Read the model definition and answer for the solid it produces. Units are mm, in the model's axes. Face numbers are marked on the shaded views. A direction names the side the tool comes from. Give positions to 0.01 mm unless a question says otherwise; leave off trailing zeros. Loops run counter-clockwise (first coordinate to the right, second up) from the corner with the lowest first, then second, coordinate; pieces in that order, holes last.
(1) Find section C-C, the plane z = 9. Write down the section's boundary in (x, y), then the cut area to 3 significant figures.
(2) Find section A-A, the plane x = -4. Write down the section's boundary in (y, z), then the cut area to 3 significant figures.
(3) Find section D-D, the plane y = 9.5. Write down the section's boundary in (x, z).
(4) Each of these flat-tipped pins is pushed along its axis until it touches: P1, Ø8, axis at y = 31, z = -1, coming from the -X side; P2, Ø5, axis at y = 30.5, z = 0, coming from the +X side; P3, Ø1, axis at x = -3, y = 29, coming from the -Z side. Where does it stop, or does it pass through?
(5) Straight lines are drawn through the part: probe 1 along X at (y, z) = (11.5, 0); probe 2 along Z at (x, y) = (-3.25, 31); probe 3 along Y at (x, z) = (-8.25, -9.5). For each, find the intervals that lie inside material, in ascending order.
(6) Which of the six approach directions +Z, -Z, +X, -X, +Y, -Y give full straight-line access (tool end or side, diameter ignored) to the marked faces 1, 2 and 3?
(7) Find section B-B, the plane x = 0. Write down the section's boundary in (y, z), then the cut area to 3 significant figures.
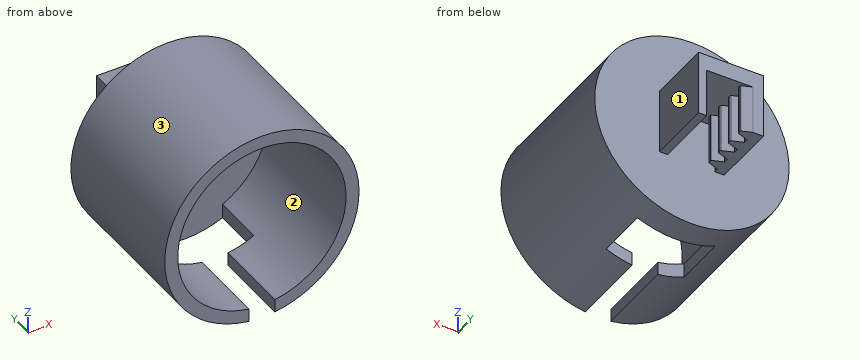
```python
from build123d import *

# Parameters (mm, degrees)
SKETCH1_R           = 15
SKETCH1_R_2         = 13
BOSS_EXTRUDE1_DEPTH = 20
SKETCH2_R           = 15
BOSS_EXTRUDE2_DEPTH = 4
SKETCH4_W           = 10
SKETCH4_H           = 10
BOSS_EXTRUDE3_DEPTH = 10
CUT_EXTRUDE2_DEPTH  = 7.5
CUT_EXTRUDE3_DEPTH  = 5


with BuildPart() as part:
    # Sketch1 → Boss-Extrude1 (new body)
    with BuildSketch(Plane(origin=(0, 0, 0), x_dir=(1, 0, 0), z_dir=(0, 1, 0))):
        with Locations(Location((0, 0, 0), (0, 0, 270))):
            Circle(SKETCH1_R)
        with Locations(Location((0, 0, 0), (0, 0, 270))):
            Circle(SKETCH1_R_2, mode=Mode.SUBTRACT)
    extrude(amount=BOSS_EXTRUDE1_DEPTH)

    # Sketch2 → Boss-Extrude2 (add)
    with BuildSketch(Plane(origin=(0, 20, 0), x_dir=(1, 0, 0), z_dir=(0, 1, 0))):
        with Locations(Location((0, 0, 0), (0, 0, 270))):
            Circle(SKETCH2_R)
    extrude(amount=BOSS_EXTRUDE2_DEPTH)

    # Sketch4 → Boss-Extrude3 (add)
    with BuildSketch(Plane(origin=(0, 24, 0), x_dir=(1, 0, 0), z_dir=(0, 1, 0))):
        Rectangle(SKETCH4_W, SKETCH4_H)
    extrude(amount=BOSS_EXTRUDE3_DEPTH)

    # Sketch6 → Cut-Extrude2 (cut)
    with BuildSketch(Plane(origin=(0, 0, -5), x_dir=(-1, 0, 0), z_dir=(0, 0, -1))):
        with BuildLine():
            Line((-1.758355149, 34), (-3.758355149, 34))
            Line((-3.758355149, 34), (-3.758355149, 24))
            Line((-3.758355149, 24), (3.541644851, 24))
            Line((3.541644851, 24), (3.541644851, 24.674283625))
            Line((3.541644851, 24.674283625), (1.891753796, 25.274794859))
            ThreePointArc((1.891753796, 25.274794859), (1.811908661, 25.336062186), (1.781644851, 25.432046729))
            Line((1.781644851, 25.432046729), (1.781644851, 25.755508896))
            ThreePointArc((1.781644851, 25.755508896), (1.811908661, 25.85149344), (1.891753796, 25.912760766))
            Line((1.891753796, 25.912760766), (3.541644851, 26.513272))
            Line((3.541644851, 26.513272), (3.541644851, 27.187555625))
            Line((3.541644851, 27.187555625), (1.891753796, 27.788066859))
            ThreePointArc((1.891753796, 27.788066859), (1.811908661, 27.849334186), (1.781644851, 27.945318729))
            Line((1.781644851, 27.945318729), (1.781644851, 28.268780896))
            ThreePointArc((1.781644851, 28.268780896), (1.811908661, 28.36476544), (1.891753796, 28.426032766))
            Line((1.891753796, 28.426032766), (3.541644851, 29.026544))
            Line((3.541644851, 29.026544), (3.541644851, 29.700827625))
            Line((3.541644851, 29.700827625), (1.891753796, 30.301338859))
            ThreePointArc((1.891753796, 30.301338859), (1.811908661, 30.362606186), (1.781644851, 30.458590729))
            Line((1.781644851, 30.458590729), (1.781644851, 30.782052896))
            ThreePointArc((1.781644851, 30.782052896), (1.811908661, 30.87803744), (1.891753796, 30.939304766))
            Line((1.891753796, 30.939304766), (3.541644851, 31.539816))
            Line((3.541644851, 31.539816), (3.541644851, 32.214099625))
            Line((3.541644851, 32.214099625), (1.891753796, 32.814610859))
            ThreePointArc((1.891753796, 32.814610859), (1.811908661, 32.875878186), (1.781644851, 32.971862729))
            Line((1.781644851, 32.971862729), (1.781644851, 33.295324896))
            ThreePointArc((1.781644851, 33.295324896), (1.811908661, 33.39130944), (1.891753796, 33.452576766))
            Line((1.891753796, 33.452576766), (3.39578677, 34))
            Line((3.39578677, 34), (0.241644851, 34))
            Line((0.241644851, 34), (-1.758355149, 34))
        make_face()
    extrude(amount=-CUT_EXTRUDE2_DEPTH, mode=Mode.SUBTRACT)

    # Sketch8 → Cut-Extrude3 (cut)
    with BuildSketch(Plane(origin=(0, 0, -15), x_dir=(-1, 0, 0), z_dir=(0, 0, -1))):
        Polygon((-6, 12), (-2, 12), (-2, 0), (2, 0), (2, 12), (6, 12), (6, 20), (-6, 20), align=None)
    extrude(amount=-CUT_EXTRUDE3_DEPTH, mode=Mode.SUBTRACT)


solid = part.part
```
Entries:
1. outline: (-12, 0) - (-9.38, 0) - (-9.38, 20) - (9.38, 20) - (9.38, 0) - (12, 0) - (12, 24) - (-12, 24) - close
1. area: 201 mm2
2. outline: (0, -14.46) - (12, -14.46) - (12, -12.37) - (0, -12.37) - close; (0, 12.37) - (20, 12.37) - (20, -14.46) - (24, -14.46) - (24, -5) - (34, -5) - (34, 5) - (24, 5) - (24, 14.46) - (0, 14.46) - close
2. area: 282 mm2
3. outline: (-2, -14.87) - (-2, -12.85) arc R13 cw (long way) to (2, -12.85) - (2, -14.87) arc R15 ccw (long way) to start
4. P1: stops at x = -5
4. P2: stops at x = 5
4. P3: stops at z = -5
5. probe 1: x = -15 to -13, 13 to 15
5. probe 2: z = -5 to 5
5. probe 3: y = 20 to 24
6. face 1: +Z, -Z, +X, +Y
6. face 2: -Y
6. face 3: +Y, -Y
7. outline: (0, 13) - (20, 13) - (20, -15) - (24, -15) - (24, 2.5) - (34, 2.5) - (34, 5) - (24, 5) - (24, 15) - (0, 15) - close
7. area: 185 mm2
